Verification items for the finished model (mm, model axes). A direction names the side the tool comes from. Round coordinates to 2 decimals unless told otherwise and drop trailing zeros. Order: outer loops, then holes, each group sorted by start corner. A loop starts at its lowest first (then second) coordinate and runs counter-clockwise, first axis right, second up. Notation, with made-up numbers: (-37, 39) -> (-24, 39) arc R20 ccw to (-24, 74) -> close; hole circle Ø9 at (9, 7). An arc over 180 degrees is marked (long way). Return JSON: item names as keys, results as strings. Group by question number.
1) Scan lines: L1, parallel to Z at x = -138.5, y = 0; L2, parallel to Y at x = -49, z = 0; L3, parallel to Y at x = -14, z = 27. Record each from-to range of solid material in increasing order.
2) Tool access check on faces 3 (the flat face through (-13, -10, 27)), 4 (the flat face through (30, 0, 72)), 5 (the flat face through (-118, 35, 69)), 6 (the flat face through (-270, 0, 72)). Record the directions out of +Z, -Z, +X, -X, +Y, -Y that give a thin tool (end or side, any length) a straight path to the whole face; none if there is none.
3) Section check A-A on y = 0. Enter the section's corners in (x, z).
4) Section check C-C on x = -145.5. Enter the section's corners in (y, z), plus the area to 3 significant figures.
5) Section check B-B on z = 63. Enter the section's corners in (x, y) (3 decimals).
6) Depth check by flat-ended pin: pin 1 (5 mm diameter, centred on y = 5, z = 31, fed in from -X); pin 2 (5 mm diameter, centred on x = -19.5, z = 22, fed in from -Y); pin 3 (1 mm diameter, centred on x = -236.5, z = 63, fed in from +Y). Enter the tip coordinate at first touch or a pass-through.
7) Draft check along Y on faces 1 (the flat face through (-11, 15, 23)), 2 (the flat face through (-300, 37, -88)). Enter one of: pulls with the +Y half, pulls with the -Y half, needs draft (parallel to the pull), parting line crosses it, or undercut.
8) Section check D-D on z = 0. Enter the section's corners in (x, y).
```python
from build123d import *

# Parameters (mm, degrees)
SKETCH_1_W           = 300
SKETCH_1_H           = 100
SKETCH_2_R           = 95
CUT_EXTRUDE_1_DEPTH  = 332.662479036
EXTRUDE_START        = 60
SKETCH_5_R           = 100
SKETCH_5_R_2         = 95
EXTRUDE_1_DEPTH      = 60
SKETCH_6_W           = 280
SKETCH_6_H           = 50
CUT_EXTRUDE_2_DEPTH  = 10
EXTRUDE_3_DEPTH      = 290
EXTRUDE_3_DEPTH_BACK = 10
SKETCH_14_W          = 300
SKETCH_14_H          = 70
EXTRUDE_5_DEPTH      = 60
SKETCH_13_W          = 280
SKETCH_13_H          = 50
CUT_EXTRUDE_3_DEPTH  = 65
FILLET_1_R           = 20
EXTRUDE_6_DEPTH      = 10
SKETCH_16_W          = 36
SKETCH_16_H          = 20
CUT_EXTRUDE_4_DEPTH  = 10
SKETCH_17_R          = 28.835
CUT_EXTRUDE_5_DEPTH  = 344.838624939


with BuildPart() as part:
    # 草图1 → 旋转1 (revolve)
    with BuildSketch(Plane(origin=(0, 0, 0), x_dir=(1, 0, 0), z_dir=(0, 1, 0)), mode=Mode.PRIVATE) as revolve_1_sk:
        with Locations((-150, -50)):
            Rectangle(SKETCH_1_W, SKETCH_1_H)
    revolve(revolve_1_sk.sketch.rotate(Axis((0, 0, 0), (-1, 0, 0)), 180), axis=Axis((0, 0, 0), (-1, 0, 0)))

    # 草图2 → 切除-拉伸1 (cut, through all)
    with BuildSketch(Plane(origin=(0, 0, 0), x_dir=(0, 0, -1), z_dir=(1, 0, 0))):
        Circle(SKETCH_2_R)
    extrude(amount=-CUT_EXTRUDE_1_DEPTH, mode=Mode.SUBTRACT)

    # 草图5 → 凸台-拉伸1 (add)
    with BuildSketch(Plane(origin=(0, 0, 0), x_dir=(0, 0, -1), z_dir=(1, 0, 0)).offset(EXTRUDE_START)):
        Circle(SKETCH_5_R)
        Circle(SKETCH_5_R_2, mode=Mode.SUBTRACT)
    extrude(amount=-EXTRUDE_1_DEPTH)

    # 草图6 → 切除-拉伸2 (cut)
    with BuildSketch(Plane.XY.offset(100)):
        with Locations((-120, 0)):
            Rectangle(SKETCH_6_W, SKETCH_6_H)
    extrude(amount=-CUT_EXTRUDE_2_DEPTH, mode=Mode.SUBTRACT)

    # 草图9 → 凸台-拉伸3 (add, two sides: drawn at the far end of the back side and taken through both)
    with BuildSketch(Plane.ZY.offset(-20).offset(-EXTRUDE_3_DEPTH_BACK)):
        with BuildLine():
            Line((88.317608663, 35), (88.317608663, -35))
            ThreePointArc((88.317608663, -35), (95, 0), (88.317608663, 35))
        make_face()
    extrude(amount=EXTRUDE_3_DEPTH + EXTRUDE_3_DEPTH_BACK)

    # 草图14 → 凸台-拉伸5 (add)
    with BuildSketch(Plane(origin=(0, 0, 88.317608663), x_dir=(-1, 0, 0), z_dir=(0, 0, -1))):
        with Locations((120, 0)):
            Rectangle(SKETCH_14_W, SKETCH_14_H)
    extrude(amount=EXTRUDE_5_DEPTH)

    # 草图13 → 切除-拉伸3 (cut)
    with BuildSketch(Plane.XY.offset(100)):
        with Locations((-120, 0)):
            Rectangle(SKETCH_13_W, SKETCH_13_H)
    extrude(amount=-CUT_EXTRUDE_3_DEPTH, mode=Mode.SUBTRACT)

    # 圆角1
    fillet_1_edges = [part.edges().sort_by_distance(p)[0] for p in [
        (-270, 0, 28.317608663),
        (-120, 35, 28.317608663),
        (30, 0, 28.317608663),
        (-120, -35, 28.317608663),
        (-260, 0, 35),
        (20, 0, 35),
    ]]
    fillet(fillet_1_edges, radius=FILLET_1_R)

    # 草图15 → 凸台-拉伸6 (add)
    with BuildSketch(Plane(origin=(0, 0, 28.317608663), x_dir=(-1, 0, 0), z_dir=(0, 0, -1))):
        Polygon((-4.931797057, -10), (-4.931797057, 10), (31.068202943, 10), (31, 15), (-4.931797057, 15), (-10, 15), (-10, 10), (-10, -10), (-10, -15), (-4.931797057, -15), (31, -15), (31.068202943, -10), align=None)
    extrude(amount=EXTRUDE_6_DEPTH)

    # 草图16 → 切除-拉伸4 (cut)
    with BuildSketch(Plane(origin=(0, 0, 28.317608663), x_dir=(-1, 0, 0), z_dir=(0, 0, -1))):
        with Locations((13.068202943, 0)):
            Rectangle(SKETCH_16_W, SKETCH_16_H)
    extrude(amount=-CUT_EXTRUDE_4_DEPTH, mode=Mode.SUBTRACT)

    # 草图17 → 切除-拉伸5 (cut, through all)
    with BuildSketch(Plane(origin=(0, 0, 35), x_dir=(-1, 0, 0), z_dir=(0, 0, -1))):
        with Locations((29.4, 0)):
            Circle(SKETCH_17_R)
    extrude(amount=-CUT_EXTRUDE_5_DEPTH, mode=Mode.SUBTRACT)


solid = part.part
```
Check result:
{
 "1": {"L1": "-100 to -95, 28.32 to 35", "L2": "-100 to -95, 95 to 100", "L3": "-96.29 to -91.08, -15 to -10, 10 to 15, 91.08 to 96.29"},
 "2": {"face 3": "+Z", "face 4": "+X", "face 5": "+X, -X", "face 6": "-X"},
 "3": {"outline": "(-300, -100) -> (60, -100) -> (60, -95) -> (-300, -95) -> close; (-300, 95) -> (-270, 95) -> (-270, 48.32) arc R20 ccw to (-250, 28.32) -> (-31.07, 28.32) -> (-31.07, 35) -> (-240, 35) arc R20 cw to (-260, 55) -> (-260, 100) -> (-300, 100) -> close; (4.93, 18.32) -> (10, 18.32) -> (10, 28.32) arc R20 ccw to (30, 48.32) -> (30, 95) -> (60, 95) -> (60, 100) -> (20, 100) -> (20, 55) arc R20 cw to (4.93, 35.62) -> close"},
 "4": {"outline": "(-25, 35) -> (-25, 96.82) arc R100 ccw (long way) to (25, 96.82) -> (25, 35) -> close; hole (-35, 48.32) -> (-35, 88.32) arc R95 ccw (long way) to (35, 88.32) -> (35, 48.32) arc R20 cw to (15, 28.32) -> (-15, 28.32) arc R20 cw to start", "area": "4,210 mm^2"},
 "5": {"outline": "(-300, -77.66) -> (60, -77.66) -> (60, -71.106) -> (-300, -71.106) -> close; (-300, 71.106) -> (60, 71.106) -> (60, 77.66) -> (-300, 77.66) -> close; (-270, -35) -> (30, -35) -> (30, 35) -> (-270, 35) -> close; hole (-260, -25) -> (-43.769, -25) arc R28.835 ccw to (-15.031, -25) -> (20, -25) -> (20, 25) -> (-15.031, 25) arc R28.835 ccw to (-43.769, 25) -> (-260, 25) -> close"},
 "6": {"pin 1": "x = -263.43", "pin 2": "y = -98.08", "pin 3": "y = 78.06"},
 "7": {"face 1": "undercut", "face 2": "needs draft"},
 "8": {"outline": "(-300, -100) -> (60, -100) -> (60, -95) -> (-300, -95) -> close; (-300, 95) -> (60, 95) -> (60, 100) -> (-300, 100) -> close"}
}
